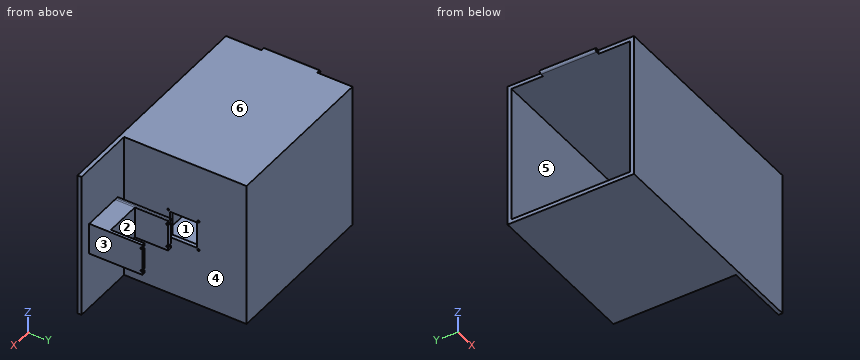
```python
from build123d import *
from build123d.topology import SkipClean

# Parameters (mm, degrees)
SKETCH1_W           = 420
SKETCH1_H           = 370
SKETCH1_W_2         = 400
SKETCH1_H_2         = 350
BOSS_EXTRUDE1_DEPTH = 300
BOSS_EXTRUDE2_DEPTH = 10
SKETCH3_W           = 10
SKETCH3_H           = 310
CUT_EXTRUDE1_DEPTH  = 370
SKETCH6_R           = 2.5
SKETCH6_W           = 68
SKETCH6_H           = 68
CUT_EXTRUDE3_DEPTH  = 10
SKETCH7_W           = 5
SKETCH7_H           = 80
BOSS_EXTRUDE3_DEPTH = 134.5
CUT_EXTRUDE4_REACH  = 646.845
SKETCH9_W           = 5
SKETCH9_H           = 79.931817825
BOSS_EXTRUDE4_DEPTH = 134.5
CUT_EXTRUDE5_REACH  = 516.637
SKETCH10_W          = 6.47899954
SKETCH10_H          = 82.791783562
SKETCH11_W          = 5
SKETCH11_H          = 80
BOSS_EXTRUDE5_DEPTH = 134.5
SKETCH12_W          = 92.5
SKETCH12_H          = 80
BOSS_EXTRUDE6_DEPTH = 50
CUT_EXTRUDE6_START  = -7.5
CUT_EXTRUDE6_DEPTH  = 105
SKETCH15_W          = 410
SKETCH15_H          = 370
BOSS_EXTRUDE7_DEPTH = 10
SKETCH16_W          = 15
SKETCH16_H          = 140.878076228
BOSS_EXTRUDE8_DEPTH = 10
SKETCH17_R          = 3
CUT_EXTRUDE7_DEPTH  = 140.878076229


with BuildPart() as part:
    # Sketch1 → Boss-Extrude1 (new body)
    with BuildSketch(Plane(origin=(0, 0, 0), x_dir=(1, 0, 0), z_dir=(0, 1, 0))):
        Rectangle(SKETCH1_W, SKETCH1_H)
        Rectangle(SKETCH1_W_2, SKETCH1_H_2, mode=Mode.SUBTRACT)
    extrude(amount=BOSS_EXTRUDE1_DEPTH)

    # Sketch2 → Boss-Extrude2 (add)
    with BuildSketch(Plane.XZ):
        Polygon((-210, -185), (210, -185), (215.001407023, -185), (375.001407023, -185), (375.001407023, 185), (215.001407023, 185), (210, 185), (-210, 185), align=None)
    extrude(amount=BOSS_EXTRUDE2_DEPTH)

    # Sketch3 → Cut-Extrude1 (cut)
    with BuildSketch(Plane.XY.offset(185)):
        with Locations((-205, 145)):
            Rectangle(SKETCH3_W, SKETCH3_H)
    extrude(amount=-CUT_EXTRUDE1_DEPTH, mode=Mode.SUBTRACT)

    # Sketch6 → Cut-Extrude3 (cut)
    with BuildSketch(Plane(origin=(210, 0, 0), x_dir=(0, 0, -1), z_dir=(1, 0, 0))):
        with Locations((-38.303, 111.697)):
            Circle(SKETCH6_R)
        with Locations((38.303, 111.697)):
            Circle(SKETCH6_R)
        with Locations((38.303, 188.303)):
            Circle(SKETCH6_R)
        with Locations((-38.303, 188.303)):
            Circle(SKETCH6_R)
        with Locations((0, 150)):
            Rectangle(SKETCH6_W, SKETCH6_H)
    extrude(amount=-CUT_EXTRUDE3_DEPTH, mode=Mode.SUBTRACT)

    # Sketch7 → Boss-Extrude3 (add)
    with BuildSketch(Plane(origin=(0, 0, 0), x_dir=(1, 0, 0), z_dir=(0, 1, 0))):
        with Locations((237.5, 0)):
            Rectangle(SKETCH7_W, SKETCH7_H)
        with Locations((337.5, 0)):
            Rectangle(SKETCH7_W, SKETCH7_H)
    extrude(amount=BOSS_EXTRUDE3_DEPTH)

    # Cut-Extrude4: up to this face of the body (flat: up to its plane)
    cut_extrude4_end = Plane(part.part.faces().sort_by_distance((235, 67.25, 0))[0])
    # Sketch8 → Cut-Extrude4 (cut, up to the picked face)
    with BuildSketch(Plane(origin=(340, 0, 0), x_dir=(0, 0, -1), z_dir=(1, 0, 0)), mode=Mode.PRIVATE) as cut_extrude4_sk1:
        with BuildLine():
            Line((-32.5, 136.110518), (-32.220758703, 136.631471953))
            Line((-32.220758703, 136.631471953), (-27.5, 136.631471953))
            Line((-27.5, 136.631471953), (-27.5, 132))
            ThreePointArc((-27.5, 132), (-30, 129.5), (-32.5, 132))
            Line((-32.5, 132), (-32.5, 136.110518))
        make_face()
    cut_extrude4_tool1 = split(extrude(cut_extrude4_sk1.sketch, amount=-CUT_EXTRUDE4_REACH, mode=Mode.PRIVATE), bisect_by=cut_extrude4_end, keep=Keep.BOTH, mode=Mode.PRIVATE)
    # Sketch8 → Cut-Extrude4 (cut, up to the picked face)
    with BuildSketch(Plane(origin=(340, 0, 0), x_dir=(0, 0, -1), z_dir=(1, 0, 0)), mode=Mode.PRIVATE) as cut_extrude4_sk2:
        with BuildLine():
            Line((27.5, 132), (27.5, 136.631471953))
            Line((27.5, 136.631471953), (32.220758703, 136.631471953))
            Line((32.220758703, 136.631471953), (32.5, 136.110518))
            Line((32.5, 136.110518), (32.5, 132))
            ThreePointArc((32.5, 132), (30, 129.5), (27.5, 132))
        make_face()
    cut_extrude4_tool2 = split(extrude(cut_extrude4_sk2.sketch, amount=-CUT_EXTRUDE4_REACH, mode=Mode.PRIVATE), bisect_by=cut_extrude4_end, keep=Keep.BOTH, mode=Mode.PRIVATE)
    add(cut_extrude4_tool1.solids().sort_by(Axis((340, 133.303425, 29.994679), (-1, 0, 0)))[0], mode=Mode.SUBTRACT)
    add(cut_extrude4_tool2.solids().sort_by(Axis((340, 133.303425, -29.994679), (-1, 0, 0)))[0], mode=Mode.SUBTRACT)

    # Sketch9 → Boss-Extrude4 (add)
    with BuildSketch(Plane(origin=(0, 0, 0), x_dir=(1, 0, 0), z_dir=(0, 1, 0))):
        with Locations((242.5, 0.034091087)):
            Rectangle(SKETCH9_W, SKETCH9_H)
    extrude(amount=BOSS_EXTRUDE4_DEPTH)

    # Cut-Extrude5: up to this face of the body (flat: up to its plane)
    cut_extrude5_end = Plane(part.part.faces().sort_by_distance((337.5, 134.5, 0))[0])
    # Sketch10 → Cut-Extrude5 (cut, up to the picked face)
    with BuildSketch(Plane(origin=(0, 0, 0), x_dir=(1, 0, 0), z_dir=(0, 1, 0)), mode=Mode.PRIVATE) as cut_extrude5_sk1:
        with Locations((334.26050023, 1.395891781)):
            Rectangle(SKETCH10_W, SKETCH10_H)
    cut_extrude5_tool1 = split(extrude(cut_extrude5_sk1.sketch, amount=CUT_EXTRUDE5_REACH, mode=Mode.PRIVATE), bisect_by=cut_extrude5_end, keep=Keep.BOTH, mode=Mode.PRIVATE)
    add(cut_extrude5_tool1.solids().sort_by(Axis((334.2605, 0, -1.395892), (0, 1, 0)))[0], mode=Mode.SUBTRACT)

    # Sketch11 → Boss-Extrude5 (add)
    with BuildSketch(Plane(origin=(0, 0, 0), x_dir=(1, 0, 0), z_dir=(0, 1, 0))):
        with Locations((342.5, 0)):
            Rectangle(SKETCH11_W, SKETCH11_H)
    extrude(amount=BOSS_EXTRUDE5_DEPTH)

    # Sketch12 → Boss-Extrude6 (add)
    with BuildSketch(Plane(origin=(0, 0, 0), x_dir=(1, 0, 0), z_dir=(0, 1, 0))):
        with Locations((291.25, 0)):
            Rectangle(SKETCH12_W, SKETCH12_H)
    extrude(amount=BOSS_EXTRUDE6_DEPTH)

    # Sketch13 → Cut-Extrude6 (cut)
    with SkipClean():  # the faces are left unmerged after this step: merging them gives an invalid solid
        with BuildSketch(Plane.ZY.offset(-337.5).offset(CUT_EXTRUDE6_START)):
            with BuildLine():
                Line((-32.5, 132), (-32.5, 134.5))
                Line((-32.5, 134.5), (-27.5, 134.5))
                Line((-27.5, 134.5), (-27.5, 132))
                ThreePointArc((-27.5, 132), (-30, 129.5), (-32.5, 132))
            make_face()
            with BuildLine():
                Line((27.5, 132), (27.5, 134.5))
                Line((27.5, 134.5), (32.5, 134.5))
                Line((32.5, 134.5), (32.5, 132))
                ThreePointArc((32.5, 132), (30, 129.5), (27.5, 132))
            make_face()
        extrude(amount=CUT_EXTRUDE6_DEPTH, mode=Mode.SUBTRACT)
    add(part.part.scale(1), mode=Mode.REPLACE)  # the faces are merged on a copy

    # Sketch15 → Boss-Extrude7 (add)
    with BuildSketch(Plane(origin=(0, 300, 0), x_dir=(1, 0, 0), z_dir=(0, 1, 0))):
        with Locations((5, 0)):
            Rectangle(SKETCH15_W, SKETCH15_H)
    extrude(amount=BOSS_EXTRUDE7_DEPTH)

    # Sketch16 → Boss-Extrude8 (add)
    with BuildSketch(Plane.XY.offset(185)):
        with Locations((-207.5, 150)):
            Rectangle(SKETCH16_W, SKETCH16_H)
    extrude(amount=-BOSS_EXTRUDE8_DEPTH)

    # Sketch17 → Cut-Extrude7 (cut)
    with BuildSketch(Plane(origin=(0, 220.439038114, 0), x_dir=(1, 0, 0), z_dir=(0, 1, 0))):
        with Locations(Location((-207.5, -180, 0), (0, 0, 270))):
            Circle(SKETCH17_R)
        with BuildLine():
            Line((-207.5, -175), (-209.035864649, -172.521100774))
            Line((-209.035864649, -172.521100774), (-216.595230293, -172.09067426))
            Line((-216.595230293, -172.09067426), (-221.114708685, -175.883807911))
            Line((-221.114708685, -175.883807911), (-223.315292371, -184.798763984))
            Line((-223.315292371, -184.798763984), (-213.821165317, -189.967050938))
            Line((-213.821165317, -189.967050938), (-207.069572146, -188.808886591))
            Line((-207.069572146, -188.808886591), (-207.5, -185))
            ThreePointArc((-207.5, -185), (-212.5, -180), (-207.5, -175))
        make_face()
    extrude(amount=-CUT_EXTRUDE7_DEPTH, mode=Mode.SUBTRACT)


solid = part.part
```
Build history of the part. All positions in model axes, mm. Face numbers are marked on the shaded views. A direction names the side the tool comes from. Give positions to 0.01 mm unless a question says otherwise; leave off trailing zeros. Loops run counter-clockwise (first coordinate to the right, second up) from the corner with the lowest first, then second, coordinate; pieces in that order, holes last.
Item 1: Flat gauge pins, fed straight in: pin 1 (5.5 mm diameter, centred on x = 237, y = 41.5, fed in from +Z); pin 2 (5 mm diameter, centred on x = -203, z = 179.5, fed in from -Y); pin 3 (3 mm diameter, centred on y = 111.697, z = -38.303, fed in from +X). Where does each tip first touch, or does it go through?
Answers follow:
pin 1: stops at z = 40
pin 2: stops at y = 79.56
pin 3: stops at x = 345
Item 2: Slice it at B-B, the plane y = 38.5. List the corners of the cut face in (x, z).
Answers follow:
outline: (-200, -185) - (210, -185) - (210, 185) - (-200, 185) - (-200, 175) - (200, 175) - (200, -175) - (-200, -175) - close; (235, -40) - (345, -40) - (345, 40) - (245, 40) - (245, 39.93) - (240, 39.93) - (240, 40) - (235, 40) - close
Item 3: Slice it at D-D, the plane z = -101. List the corners of the cut face in (x, y), and give its area (4 significant figures).
Answers follow:
outline: (-200, -10) - (375, -10) - (375, 0) - (210, 0) - (210, 310) - (-200, 310) - (-200, 300) - (200, 300) - (200, 0) - (-200, 0) - close
area: 12,850 mm2
Item 4: Slice it at C-C, the plane x = 184.5. List the corners of the cut face in (y, z), and give its area (3 significant figures).
Answers follow:
outline: (-10, -185) - (310, -185) - (310, 185) - (-10, 185) - close; hole (0, -175) - (300, -175) - (300, 175) - (0, 175) - close
area: 13,400 mm2
Item 5: Drill centre lines: line 1 (X direction, y = 67, z = 5); line 2 (Y direction, x = 98, z = 102); line 3 (Z direction, x = 164.5, y = 168.5). Where is each one in solid material? Low to high.
Answers follow:
line 1: x = 200 to 210, 235 to 245, 337.5 to 345
line 2: y = -10 to 0, 300 to 310
line 3: z = -185 to -175, 175 to 185
Item 6: Slice it at A-A, the plane y = 94. List the corners of the cut face in (x, z).
Answers follow:
outline: (-207.5, 175) - (200, 175) - (200, -175) - (-200, -175) - (-200, -185) - (210, -185) - (210, 185) - (-207.5, 185) arc R5 ccw to start; (235, -40) - (245, -40) - (245, 39.93) - (240, 39.93) - (240, 40) - (235, 40) - close; (337.5, -40) - (345, -40) - (345, 40) - (337.5, 40) - close; hole circle Ø6 at (-207.5, 180)
Item 7: Which spindle directions (+Z, -Z, +X, -X, +Y, -Y) get a long thin tool onto all of the face, cutting with end or side? Do the marked faces 1, 2 and 3. Say none if no direction does.
Answers follow:
face 1: -X
face 2: +Z, -Z, +Y
face 3: +Z, -Z, +X, +Y
Item 8: Pull direction Z, two halves, no side cores. Call the marked faces 4, 5 and 6: released by +Z, released by -Z, zero draft, split by the parting line, or undercut.
Answers follow:
face 4: zero draft
face 5: undercut
face 6: released by +Z
